Build history of the part. All positions in model axes, mm. Coordinates: 2 decimals unless noted, no trailing zeros. Order: outer loops, then holes, each group sorted by start corner. A loop starts at its lowest first (then second) coordinate and runs counter-clockwise, first axis right, second up. Notation, with made-up numbers: (-22.5, 71.25) - (0.5, 71.25) arc R11 cw to (0.5, 87.25) - close; hole circle Ø11 at (34.25, 89.25). An arc over 180 degrees is marked (long way). Return JSON: item names as keys, results as strings.
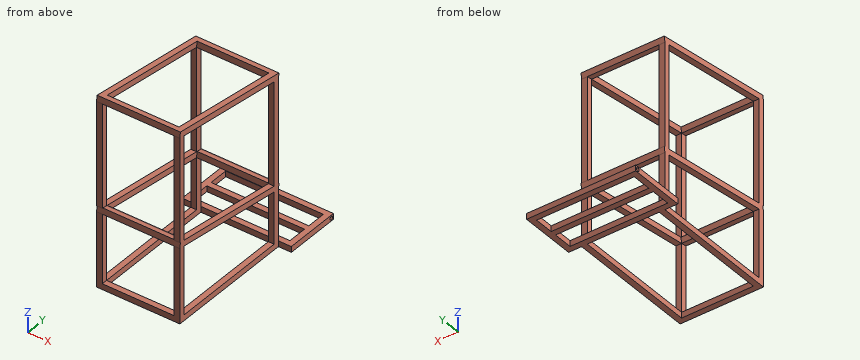
from build123d import *

# Parameters (mm, degrees)
F0_W     = 431.8
F0_H     = 25.4
F1_DEPTH = 25.4
F3_DEPTH = 25.4
F5_DEPTH = 368.3
F6_R     = 7.9375
F7_DEPTH = 482.6


with BuildPart() as f1:
    # F0 (on Top) → F1 (new body)
    with BuildSketch(Plane.XY):
        Polygon((241.3, 123.825), (-241.3, 123.825), (-241.3, -123.825), (-184.15, -123.825), (-158.75, -123.825), (158.75, -123.825), (184.15, -123.825), (241.3, -123.825), align=None)
        Polygon((-215.9, 98.425), (215.9, 98.425), (215.9, 12.7), (215.9, -12.7), (215.9, -98.425), (-215.9, -98.425), (-215.9, -12.7), (-215.9, 12.7), align=None, mode=Mode.SUBTRACT)
        Polygon((-158.75, -123.825), (-184.15, -123.825), (-184.15, -703.2752), (184.15, -703.2752), (184.15, -123.825), (158.75, -123.825), (158.75, -677.8752), (-158.75, -677.8752), align=None)
        Rectangle(F0_W, F0_H)
    extrude(amount=-F1_DEPTH)

    # F4: F3 across plane


with BuildPart() as f3:
    # F2 (on face) → F3 (new body)
    with BuildSketch(Plane.YZ.offset(184.15)):
        Polygon((-699.8117743353, 329.9627638121), (-703.2752, 304.8), (-677.8752, 301.3039209309), (-674.4117743353, 326.466684743), (-677.8752, 326.9433937971), align=None)
        Polygon((-674.4117743353, 326.466684743), (-677.8752, 301.3039209309), (-149.225, 228.5400272659), (-145.7615743353, 253.702791078), (-149.225, 254.1795001321), align=None)
        Polygon((-703.2752, 330.4394728662), (-699.8117743353, 329.9627638121), (-677.8752, 326.9433937971), (-677.8752, 783.9039209309), (-703.2752, 787.4), align=None)
        Polygon((-145.7615743353, 253.702791078), (-149.225, 228.5400272659), (-123.825, 225.0439481968), (-120.3615743353, 250.2067120089), (-123.825, 250.683421063), align=None)
        Polygon((-149.225, 254.1795001321), (-145.7615743353, 253.702791078), (-123.825, 250.683421063), (-123.825, 707.6439481968), (-149.225, 711.1400272659), align=None)
        Polygon((-674.4117743353, 809.066684743), (-677.8752, 783.9039209309), (-149.225, 711.1400272659), (-145.7615743353, 736.302791078), align=None)
        Polygon((-703.2752, 787.4), (-677.8752, 783.9039209309), (-674.4117743353, 809.066684743), (-699.8117743353, 812.5627638121), align=None)
        Polygon((-145.7615743353, 736.302791078), (-149.225, 711.1400272659), (-123.825, 707.6439481968), (-120.3615743353, 732.8067120089), align=None)
        Polygon((-703.2752, 304.8), (-703.2752, 0), (-677.8752, 0), (-677.8752, 301.3039209309), align=None)
        Polygon((-149.225, 228.5400272659), (-149.225, 0), (-123.825, 0), (-123.825, 225.0439481968), align=None)
    extrude(amount=-F3_DEPTH)


with BuildPart() as f1_1:
    add(f1.part)
    add(f3.part.mirror(Plane.YZ))


    add(f3.part)  # F5 merges F3
    # F2 (on face) → F5 (join)
    with BuildSketch(Plane.YZ.offset(184.15)):
        Polygon((-699.8117743353, 329.9627638121), (-703.2752, 304.8), (-677.8752, 301.3039209309), (-674.4117743353, 326.466684743), (-677.8752, 326.9433937971), align=None)
        Polygon((-145.7615743353, 253.702791078), (-149.225, 228.5400272659), (-123.825, 225.0439481968), (-120.3615743353, 250.2067120089), (-123.825, 250.683421063), align=None)
        Polygon((-703.2752, 787.4), (-677.8752, 783.9039209309), (-674.4117743353, 809.066684743), (-699.8117743353, 812.5627638121), align=None)
        Polygon((-145.7615743353, 736.302791078), (-149.225, 711.1400272659), (-123.825, 707.6439481968), (-120.3615743353, 732.8067120089), align=None)
    extrude(amount=-F5_DEPTH)

    # F6 (on face) → F7 (cut)
    with BuildSketch(Plane.YZ.offset(241.3)):
        with Locations((111.125, -12.7)):
            Circle(F6_R)
    extrude(amount=-F7_DEPTH, mode=Mode.SUBTRACT)


solid = f1_1.part
1. Drop flat-ended pins along their axis: pin 1 (12.5 mm diameter, centred on x = 174.5, z = 144.5, fed in from +Y) (3 decimals); pin 2 (14.5 mm diameter, centred on y = 111.125, z = -12.7, fed in from -X); pin 3 (10 mm diameter, centred on x = 174.5, y = -529, fed in from +Z); pin 4 (7.5 mm diameter, centred on x = 174, y = -393.5, fed in from +Z). Give the stop position or say it passes through.
Check values:
{"pin 1": "y = -123.825", "pin 2": "through", "pin 3": "z = 789.74", "pin 4": "z = 770.92"}
2. Cut at D-D on x = 86.5. State how many separate pieces and enclosed holes the cut face has, plus the area to 3 significant figures.
Check values:
{"separate pieces": "8", "enclosed holes": "1", "area": "4,990 mm²"}
3. Probe L1, parallel to Y at x = -181, z = 476 (3 decimals); L2, parallel to Y at x = -112, z = -12 (3 decimals); L3, parallel to Z at x = -174, y = -601. List the from-to ranges inside material, lowest first.
Check values:
{"L1": "-703.275 to -677.875, -149.225 to -123.825", "L2": "-703.275 to -677.875, -123.825 to -98.425, -12.7 to 12.7, 98.425 to 103.218, 119.032 to 123.825", "L3": "-25.4 to 0, 290.72 to 316.36, 773.32 to 798.96"}
4. Cut at B-B on y = 31. Give the cut face in (x, z), plus the area to 3 significant figures.
Check values:
{"outline": "(-241.3, -25.4) - (-215.9, -25.4) - (-215.9, 0) - (-241.3, 0) - close; (215.9, -25.4) - (241.3, -25.4) - (241.3, 0) - (215.9, 0) - close", "area": "1,290 mm²"}
5. Cut at C-C on z = 458. Give the cut face in (x, y) (3 decimals), plus the area to 3 significant figures.
Check values:
{"outline": "(-184.15, -703.275) - (-158.75, -703.275) - (-158.75, -677.875) - (-184.15, -677.875) - close; (-184.15, -149.225) - (-158.75, -149.225) - (-158.75, -123.825) - (-184.15, -123.825) - close; (158.75, -703.275) - (184.15, -703.275) - (184.15, -677.875) - (158.75, -677.875) - close; (158.75, -149.225) - (184.15, -149.225) - (184.15, -123.825) - (158.75, -123.825) - close", "area": "2,580 mm²"}
6. Cut at A-A on x = 197. Give the cut face in (y, z) (1 decimal).
Check values:
{"outline": "(-123.8, -25.4) - (-98.4, -25.4) - (-98.4, 0) - (-123.8, 0) - close; (-12.7, -25.4) - (12.7, -25.4) - (12.7, 0) - (-12.7, 0) - close; (98.4, -25.4) - (123.8, -25.4) - (123.8, 0) - (98.4, 0) - close; hole circle Ø15.9 at (111.1, -12.7)"}
